CAD build for the part. Positions are in the model's coordinates, mm. Give positions to 0.01 mm unless a question says otherwise; leave off trailing zeros. Loops run counter-clockwise (first coordinate to the right, second up) from the corner with the lowest first, then second, coordinate; pieces in that order, holes last. Notation, with made-up numbers: (-17.75, 73.5) -> (-9.75, 73.5) arc R24 cw to (-9.75, 106.5) -> close; hole circle Ø4 at (5.5, 68). An arc over 180 degrees is marked (long way). Use one line per item in the form item = value.
Autodesk Inventor part; units mm, degrees
ref_plane "YZ Plane" through (0, 0, 0) normal (1, 0, 0) x (0, 1, 0)
ref_plane "XZ Plane" through (0, 0, 0) normal (0, 1, 0) x (-1, 0, 0)
ref_plane "XY Plane" through (0, 0, 0) normal (0, 0, 1) x (1, 0, 0)
sketch "Sketch1" plane through (0, 0, 0) normal (0, 0, 1) x (1, 0, 0)
  circle A0 centre (0, 0) radius 14.2875
  circle A1 centre (-25.4, 41.275) radius 2.0701
  circle A2 centre (0, 41.275) radius 2.0701
  circle A3 centre (25.4, 41.275) radius 2.0701
  line L0 (-25.4, 41.275) -> (25.4, 41.275) construction
  circle A4 centre (0, 0) radius 22.225
  line L1 (-25.4, 41.275) -> (25.4, 41.275) construction
  line L2 (-25.4, 28.575) -> (25.4, 28.575) construction
  line L3 (25.4, 53.975) -> (-25.4, 53.975)
  arc A5 (-25.4, 53.975) -> (-25.4, 28.575) centre (-25.4, 41.275) ccw
  arc A6 (25.4, 28.575) -> (25.4, 53.975) centre (25.4, 41.275) ccw
  line L4 (-20.8482, -7.7008) -> (-37.3133, 36.8745)
  line L5 (1.8331, -22.86) -> (-1.8331, -22.86) construction
  line L6 (-1.8331, -22.86) -> (-3.6662, -19.685) construction
  line L7 (-3.6662, -19.685) -> (-1.8331, -16.51) construction
  line L8 (-1.8331, -16.51) -> (1.8331, -16.51) construction
  line L9 (1.8331, -16.51) -> (3.6662, -19.685) construction
  line L10 (3.6662, -19.685) -> (1.8331, -22.86) construction
  circle A7 centre (0, 0) radius 16.51 construction
  circle A8 centre (0, -19.685) radius 2.0701
  line L11 (0, -19.685) -> (0, 0) construction
  circle A9 centre (0, -19.685) radius 5.3975
  arc A10 (-4.2797, -22.9739) -> (-6.8869, -21.1311) centre (-8.5594, -26.2629) ccw
  arc A11 (6.8869, -21.1311) -> (4.2797, -22.9739) centre (8.5594, -26.2629) ccw
  circle A12 centre (0, -19.685) radius 4.0005 construction
  line L12 (20.8482, -7.7008) -> (37.3133, 36.8745)
  point P0 (0, -22.86)
  dimension "d0" = 25.4
  dimension "d4" = 4.1402
  dimension "d5" = 28.575
  dimension "d6" = 44.45
  dimension "d7" = 25.4
  dimension "d10" = 6.35
  dimension "d11" = 33.02
  dimension "d12" = 8.001
  dimension "d13" = 41.275
extrude "Extrusion1" add sketch "Sketch1" along normal blind 3.175
sketch "Sketch2" plane through (0, 0, 3.175) normal (0, 0, 1) x (1, 0, 0)
  arc A0 (-4.2797, -22.9739) -> (-6.8869, -21.1311) centre (-8.5594, -26.2629) ccw
  arc A1 (-4.2797, -22.9739) -> (4.2797, -22.9739) centre (0, -19.685) ccw
  arc A2 (6.8869, -21.1311) -> (4.2797, -22.9739) centre (8.5594, -26.2629) ccw
  arc A3 (6.8869, -21.1311) -> (20.8482, -7.7008) centre (0, 0) ccw
  line L0 (20.8482, -7.7008) -> (37.3133, 36.8745)
  arc A4 (37.3133, 36.8745) -> (25.4, 53.975) centre (25.4, 41.275) ccw
  line L1 (25.4, 53.975) -> (-25.4, 53.975)
  arc A5 (-25.4, 53.975) -> (-37.3133, 36.8745) centre (-25.4, 41.275) ccw
  line L2 (-37.3133, 36.8745) -> (-20.8482, -7.7008)
  arc A6 (-20.8482, -7.7008) -> (-6.8869, -21.1311) centre (0, 0) ccw
  circle A7 centre (0, 0) radius 14.2875
  circle A8 centre (0, -19.685) radius 2.0701
  circle A9 centre (0, 41.275) radius 2.0701
  circle A10 centre (25.4, 41.275) radius 2.0701
  circle A11 centre (-25.4, 41.275) radius 2.0701
properties part number "Intake Motor Holder Using 1__16 Gray Tinted Polycarbonate Sheet (36 x 72) (217-6627)" material "Polycarbonate, Clear"
1. Mould opens along X. For faces 1 (the cylindrical face through (-35.92, 48.39, 1.57)), 2 (the cylindrical face through (-27.043, 42.535, 1.565)), 3 (the flat face through (28.965, 14.275, 1.565)) say: pulls with the +X half, pulls with the -X half, needs draft (parallel to the pull), parting line crosses it, or undercut.
Result sheet:
face_1 = pulls with the -X half
face_2 = undercut
face_3 = pulls with the +X half
2. Cut at B-B, the plane x = 9. Write the cut outline in (y, z) (3 decimals), then the cut area to 3 significant figures.
Result sheet:
outline = (-20.321, 0) -> (-11.097, 0) -> (-11.097, 3.175) -> (-20.321, 3.175) -> close; (11.097, 0) -> (53.975, 0) -> (53.975, 3.175) -> (11.097, 3.175) -> close
area = 165 mm^2
3. Cut at D-D, the plane z = 1.8. State how many separate pieces and enclosed holes the cut face has, then the cut area to 3 significant figures.
Result sheet:
separate_pieces = 1
enclosed_holes = 5
area = 3,590 mm^2
4. Cut at A-A, the plane x = 0. Write the cut outline in (y, z) (1 decimal), then the cut area to 3 significant figures.
Result sheet:
outline = (-25.1, 0) -> (-21.8, 0) -> (-21.8, 3.2) -> (-25.1, 3.2) -> close; (-17.6, 0) -> (-14.3, 0) -> (-14.3, 3.2) -> (-17.6, 3.2) -> close; (14.3, 0) -> (39.2, 0) -> (39.2, 3.2) -> (14.3, 3.2) -> close; (43.3, 0) -> (54, 0) -> (54, 3.2) -> (43.3, 3.2) -> close
area = 134 mm^2
5. Drill centre lines: line 1 (X direction, y = 41, z = 1.9); line 2 (X direction, y = -8.5, z = 1.65); line 3 (X direction, y = -10.5, z = 1.8). Where is each one in solid material? Low to high.
Result sheet:
line_1 = -38.1 to -27.45, -23.35 to -2.05, 2.05 to 23.35, 27.45 to 38.1
line_2 = -20.54 to -11.48, 11.48 to 20.54
line_3 = -19.59 to -9.69, 9.69 to 19.59
6. Cut at C-C, the plane y = 0. Write the cut outline in (x, z) (1 decimal), then the cut area to 3 significant figures.
Result sheet:
outline = (-23.7, 0) -> (-14.3, 0) -> (-14.3, 3.2) -> (-23.7, 3.2) -> close; (14.3, 0) -> (23.7, 0) -> (23.7, 3.2) -> (14.3, 3.2) -> close
area = 59.7 mm^2
